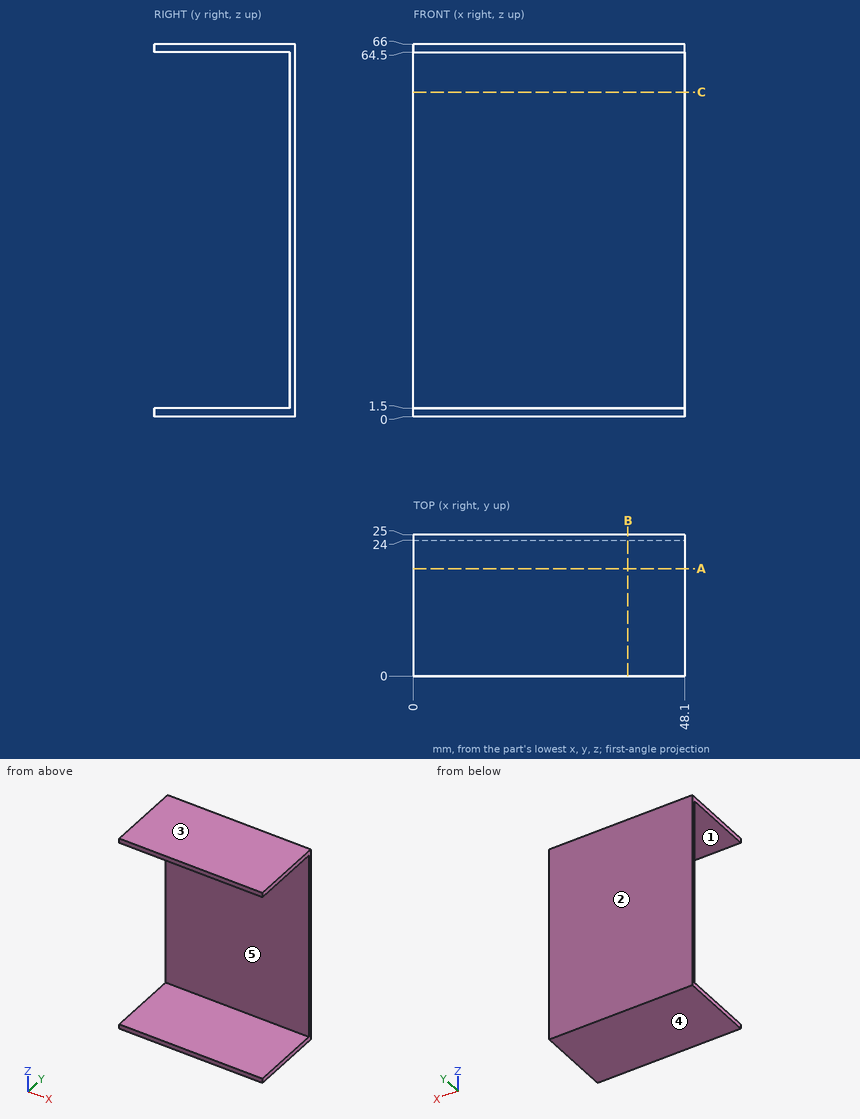
Here's the drawing with two shaded views (mm, measured from the low corner). I have some questions. A direction names the side the tool comes from. Coordinates: 2 decimals unless noted, no trailing zeros. Write each loop counter-clockwise with the first axis right and the second up, starting at its lowest first coordinate (ties: lowest second). Pieces come first, ordered by that corner, then holes. Notation, with made-up numbers: (36, -4.5) -> (66, -4.5) arc R27 cw to (66, 27.5) -> close; hole circle Ø2 at (89.5, 33.5). An arc over 180 degrees is marked (long way). One line per question, with ' | ' between items. Start each with the question number.
1. If we section it at B-B (x = 38): Please give me the cut outline in (y, z), and give its area (3 significant figures).
2. If we section it at A-A (y = 19): Please give me the cut outline in (x, z), and give its area (3 significant figures).
3. Thinking about a two-plate mould opening in Z: for the marked faces 3, 4 and 5, which applies, pulls with the +Z half, pulls with the -Z half, needs draft (parallel to the pull), parting line crosses it, or undercut?
4. For the marked faces 1 and 2, which set-ups out of +Z, -Z, +X, -X, +Y, -Y let a thin tool reach every point of the face, with its end or its side?
5. Will this pin go through, and if not, where does the flat tip stop? P1, Ø24, axis at x = 34.5, z = 23, coming from the -Y side.
6. Please list where these lines run through material, in increasing order: line 1 along Z through (x, y) = (6, 8); line 2 along Y through (x, z) = (10.5, 53.5).
7. If we section it at C-C (z = 57.5): Please give me the cut outline in (x, y), and give its area (3 significant figures).
Return value:
1) outline: (0, 0) -> (25, 0) -> (25, 66) -> (0, 66) -> (0, 64.5) -> (24, 64.5) -> (24, 1.5) -> (0, 1.5) -> close | area: 138 mm²
2) outline: (0, 0) -> (48.1, 0) -> (48.1, 1.5) -> (0, 1.5) -> close; (0, 64.5) -> (48.1, 64.5) -> (48.1, 66) -> (0, 66) -> close | area: 144 mm²
3) face 3: pulls with the +Z half | face 4: pulls with the -Z half | face 5: undercut
4) face 1: +X, -X, -Y | face 2: +Z, -Z, +X, -X, +Y
5) P1: stops at y = 24
6) line 1: z = 0 to 1.5, 64.5 to 66 | line 2: y = 24 to 25
7) outline: (0, 24) -> (48.1, 24) -> (48.1, 25) -> (0, 25) -> close | area: 48.1 mm²
